Design review of the part built by this model. Coordinates are the model's own, in mm. A direction names the side the tool comes from. Round coordinates to 2 decimals unless told otherwise and drop trailing zeros. Order: outer loops, then holes, each group sorted by start corner. A loop starts at its lowest first (then second) coordinate and runs counter-clockwise, first axis right, second up. Notation, with made-up numbers: M -30.5,15 L 10.5,15 A12 cw 10.5,22 Z; hole C 7.5,2 d3. An arc over 180 degrees is marked long. Use a Markdown table: item, result. Add a question column.
(1) For pin 1 (1.6 mm diameter, centred on x = 0, z = 0, fed in from -Y); pin 2 (1.2 mm diameter, centred on y = 3.5, z = -0.5, fed in from +X); pin 3 (2 mm diameter, centred on y = 3.5, z = 0, fed in from -X); pin 4 (2 mm diameter, centred on x = -3.5, z = 1, fed in from +Y), all flat-tipped, find the tip position at first contact; note any pin that passes through.
(2) Take a section at A-A (z = 0). Write out the cut boundary in (x, y) (3 decimals).
(3) To check wall thickness, follow probe 1 along X at (y, z) = (3, 1.1); probe 2 along Y at (x, z) = (0, 1.75); probe 3 along Y at (x, z) = (-2, -1.5). State the ranges of each line that lie inside material, in increasing order. Write a range as from..to.
(4) Machinability: for faces 4 (the face through (-6, 1, 0.5)), 5 (the face through (5.42, 1.03, -1.24)), 6 (the face through (-3.758, -0.068, -1.24)), which of the approach directions +Z, -Z, +X, -X, +Y, -Y give a long, thin tool a straight path to every point of the face, cutting with its end or side? Answer none if there is none.
(5) Take a section at C-C (x = 4.75). Write out the cut boundary in (y, z).
(6) Take a section at B-B (y = 2.5). Write out the cut boundary in (x, z).
(7) Take a section at D-D (y = -0.5). Write out the cut boundary in (x, z).
(8) The part is to be moulded in two halves that separate along X. For faces 1 (the face through (6, 1, 0.5)), 2 (the face through (5, 4, 0)), 3 (the face through (5.42, 1.03, 1.26)), say which applies: released by +X, released by -X, zero draft, split by the parting line, or undercut.
```python
from build123d import *

# Parameters (mm, degrees)
SKETCH1_R               = 0.15
BOSS_EXTRUDE1_DEPTH     = 2
BOSS_EXTRUDE3_DEPTH     = 0.5
CUT_EXTRUDE1_DEPTH      = 9.910022596
CUT_EXTRUDE1_DEPTH_BACK = 9.910022596
CUT_EXTRUDE2_DEPTH      = 4.310022596
CUT_EXTRUDE2_DEPTH_BACK = 15.510022596
SKETCH6_R               = 1
CUT_EXTRUDE3_DEPTH      = 7.43
CUT_EXTRUDE3_DEPTH_BACK = 1.953161862


with BuildPart() as part:
    # Sketch1 → Boss-Extrude1 (new body, symmetric)
    with BuildSketch(Plane.XY):
        with BuildLine():
            Line((-2.405, -0.95), (2.405, -0.95))
            ThreePointArc((2.405, -0.95), (2.440204468, -0.822082529), (2.535903035, -0.73019119))
            Line((2.535903035, -0.73019119), (4.945484826, 0.575370124))
            ThreePointArc((4.945484826, 0.575370124), (5.423977661, 1.034826819), (5.6, 1.674414174))
            Line((5.6, 1.674414174), (5.6, 6.43))
            Line((5.6, 6.43), (5, 6.43))
            Line((5, 6.43), (5, 1.58))
            Line((5, 1.58), (4.95, 1.53))
            Line((4.95, 1.53), (-4.95, 1.53))
            Line((-4.95, 1.53), (-5, 1.58))
            Line((-5, 1.58), (-5, 6.43))
            Line((-5, 6.43), (-5.6, 6.43))
            Line((-5.6, 6.43), (-5.6, 1.674414174))
            ThreePointArc((-5.6, 1.674414174), (-5.423977661, 1.034826819), (-4.945484826, 0.575370124))
            Line((-4.945484826, 0.575370124), (-2.535903035, -0.73019119))
            ThreePointArc((-2.535903035, -0.73019119), (-2.440204468, -0.822082529), (-2.405, -0.95))
        make_face()
        Circle(SKETCH1_R, mode=Mode.SUBTRACT)
    extrude(amount=BOSS_EXTRUDE1_DEPTH, both=True)

    # Sketch2 → Boss-Extrude3 (add, symmetric)
    with BuildSketch(Plane.XY):
        with BuildLine():
            Line((2.535903035, -0.73019119), (4.945484826, 0.575370124))
            ThreePointArc((4.945484826, 0.575370124), (5.423977661, 1.034826819), (5.6, 1.674414174))
            Line((5.6, 1.674414174), (5.6, 4.81))
            Line((5.6, 4.81), (8.042875866, 2.967187611))
            ThreePointArc((8.042875866, 2.967187611), (8.777798155, 0.479164908), (6.61265257, -0.95))
            Line((6.61265257, -0.95), (2.535903035, -0.73019119))
        make_face()
        with BuildLine():
            Line((-2.535903035, -0.73019119), (-4.945484826, 0.575370124))
            ThreePointArc((-4.945484826, 0.575370124), (-5.423977661, 1.034826819), (-5.6, 1.674414174))
            Line((-5.6, 1.674414174), (-5.6, 4.81))
            Line((-5.6, 4.81), (-8.042875866, 2.967187611))
            ThreePointArc((-8.042875866, 2.967187611), (-8.777798155, 0.479164908), (-6.61265257, -0.95))
            Line((-6.61265257, -0.95), (-2.535903035, -0.73019119))
        make_face()
    extrude(amount=BOSS_EXTRUDE3_DEPTH, both=True)

    # Sketch4 → Cut-Extrude1 (cut, two sides)
    with BuildSketch(Plane(origin=(0, 0, 0), x_dir=(0, 0, -1), z_dir=(1, 0, 0))) as cut_extrude1_sk:
        with BuildLine():
            Line((0.75, 5.47), (0.75, 6.97))
            Line((0.75, 6.97), (-0.75, 6.97))
            Line((-0.75, 6.97), (-0.75, 5.47))
            ThreePointArc((-0.75, 5.47), (0, 4.72), (0.75, 5.47))
        make_face()
    extrude(amount=CUT_EXTRUDE1_DEPTH, mode=Mode.SUBTRACT)
    extrude(cut_extrude1_sk.sketch, amount=-CUT_EXTRUDE1_DEPTH_BACK, mode=Mode.SUBTRACT)

    # Sketch5 → Cut-Extrude2 (cut, two sides)
    with BuildSketch(Plane(origin=(5.6, 0, 0), x_dir=(0, 0, -1), z_dir=(1, 0, 0))) as cut_extrude2_sk:
        with BuildLine():
            Line((2, 6.43), (2, 5.68))
            ThreePointArc((2, 5.68), (1.780330086, 6.210330086), (1.25, 6.43))
            Line((1.25, 6.43), (2, 6.43))
        make_face()
        with BuildLine():
            Line((-2, 6.43), (-2, 5.68))
            ThreePointArc((-2, 5.68), (-1.780330086, 6.210330086), (-1.25, 6.43))
            Line((-1.25, 6.43), (-2, 6.43))
        make_face()
    extrude(amount=CUT_EXTRUDE2_DEPTH, mode=Mode.SUBTRACT)
    extrude(cut_extrude2_sk.sketch, amount=-CUT_EXTRUDE2_DEPTH_BACK, mode=Mode.SUBTRACT)

    # Sketch6 → Cut-Extrude3 (cut, two sides)
    with BuildSketch(Plane(origin=(0, 0, 0), x_dir=(1, 0, 0), z_dir=(0, 1, 0))) as cut_extrude3_sk:
        Circle(SKETCH6_R)
    extrude(amount=CUT_EXTRUDE3_DEPTH, mode=Mode.SUBTRACT)
    extrude(cut_extrude3_sk.sketch, amount=-CUT_EXTRUDE3_DEPTH_BACK, mode=Mode.SUBTRACT)


solid = part.part
```
Verdict:
| question | item | result |
|---|---|---|
| 1 | pin 1 | passes through |
| 1 | pin 2 | stops at x = 8.13 |
| 1 | pin 3 | stops at x = -8.5 |
| 1 | pin 4 | stops at y = 1.53 |
| 2 | outline | M -8.043,2.967 A2.18 ccw -6.613,-0.95 L -2.536,-0.73 A0.25 cw -2.405,-0.95 L -1,-0.95 L -1,1.53 L -4.95,1.53 L -5,1.58 L -5,4.72 L -5.719,4.72 Z; M 1,-0.95 L 2.405,-0.95 A0.25 cw 2.536,-0.73 L 6.613,-0.95 A2.18 ccw 8.043,2.967 L 5.719,4.72 L 5,4.72 L 5,1.58 L 4.95,1.53 L 1,1.53 Z |
| 3 | probe 1 | x = -5.6..-5, 5..5.6 |
| 3 | probe 2 | y = -0.95..-0.15, 0.15..1.53 |
| 3 | probe 3 | y = -0.95..1.53 |
| 4 | face 4 | +Z, -X, -Y |
| 4 | face 5 | -Z, +X, -Y |
| 4 | face 6 | -Z, -X, -Y |
| 5 | outline | M -0.85,-0.5 L 0.47,-0.5 L 0.47,-2 L 1.53,-2 L 1.53,2 L 0.47,2 L 0.47,0.5 L -0.85,0.5 Z |
| 6 | outline | M -8.5,-0.5 L -5.6,-0.5 L -5.6,-2 L -5,-2 L -5,2 L -5.6,2 L -5.6,0.5 L -8.5,0.5 Z; M 5,-2 L 5.6,-2 L 5.6,-0.5 L 8.5,-0.5 L 8.5,0.5 L 5.6,0.5 L 5.6,2 L 5,2 Z |
| 7 | outline | M -8.06,-0.5 L -2.96,-0.5 L -2.96,-2 L 2.96,-2 L 2.96,-0.5 L 8.06,-0.5 L 8.06,0.5 L 2.96,0.5 L 2.96,2 L -2.96,2 L -2.96,0.5 L -8.06,0.5 Z; hole C 0,0 d2 |
| 8 | face 1 | zero draft |
| 8 | face 2 | undercut |
| 8 | face 3 | released by +X |
